Here's the drawing with two shaded views (mm, measured from the low corner). I have some questions. A direction names the side the tool comes from. Round coordinates to 2 decimals unless told otherwise and drop trailing zeros. Order: outer loops, then holes, each group sorted by start corner. A loop starts at its lowest first (then second) coordinate and runs counter-clockwise, first axis right, second up.
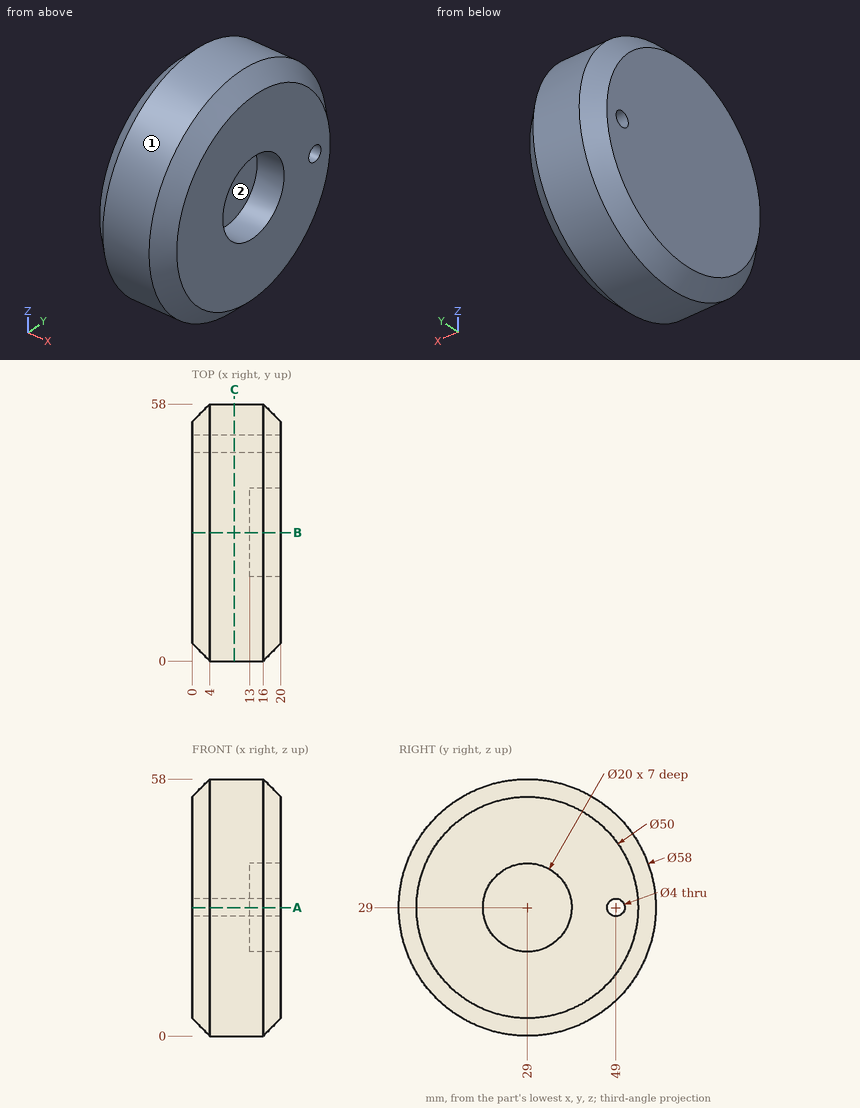
1. On a 3-axis mill with a long thin cutter (end or side, diameter ignored), from which of +Z, -Z, +X, -X, +Y, -Y can I reach the whole of each face in a straight line? I mean the marked faces 1 and 2. Say none if no direction works.
Evaluation:
face 1: +X, -X
face 2: +X
2. I'm going to push flat-ended pins straight in: P1, Ø10, axis at y = 29.5, z = 28, coming from the +X side; P2, Ø10, axis at x = 8.5, y = 13, coming from the -Z side; P3, Ø2, axis at x = 9.5, z = 18, coming from the +Y side; P4, Ø23, axis at y = 29, z = 29, coming from the +X side. Where does each tip first touch, or does it pass through?
Evaluation:
P1: stops at x = 13
P2: stops at z = 2.17
P3: stops at y = 56.22
P4: stops at x = 20
3. If we section it at B-B, the plane y = 29: Write out the boundary of the cut face in (x, z), and give its area (3 significant figures).
Evaluation:
outline: (0, 4) - (4, 0) - (16, 0) - (20, 4) - (20, 19) - (13, 19) - (13, 39) - (20, 39) - (20, 54) - (16, 58) - (4, 58) - (0, 54) - close
area: 988 mm2
4. If we section it at A-A, the plane z = 29: Write out the boundary of the cut face in (x, y), and give its area (3 significant figures).
Evaluation:
outline: (0, 4) - (4, 0) - (16, 0) - (20, 4) - (20, 19) - (13, 19) - (13, 39) - (20, 39) - (20, 47) - (0, 47) - close; (0, 51) - (20, 51) - (20, 54) - (16, 58) - (4, 58) - (0, 54) - close
area: 908 mm2
5. If we section it at C-C, the plane x = 9.5: Write out the boundary of the cut face in (y, z), and give its area (3 significant figures).
Evaluation:
outline: circle Ø58 at (29, 29); hole circle Ø4 at (49, 29)
area: 2,630 mm2
6. I need wall thicknesses on probe 1 along Y at (x, z) = (15, 29); probe 2 along Y at (x, z) = (12.5, 29); probe 3 along X at (y, z) = (23.5, 36.5). Which ranges of each line are inside material? Lowest first, please.
Evaluation:
probe 1: y = 0 to 19, 39 to 47, 51 to 58
probe 2: y = 0 to 47, 51 to 58
probe 3: x = 0 to 13
